```python
from build123d import *

# Parameters (mm, degrees)
SKETCH_R     = 16.037804
SKETCH_R_2   = 13.697081
PAD_DEPTH    = 50
POCKET_DEPTH = 18


with BuildPart() as part:
    # Sketch → Pad (new body)
    with BuildSketch(Plane.XZ):
        Circle(SKETCH_R)
        Circle(SKETCH_R_2, mode=Mode.SUBTRACT)
    extrude(amount=PAD_DEPTH)

    # Sketch001 → Pocket (cut)
    with BuildSketch(Plane.XY):
        Polygon((8.285895, -29.05966), (9.186356, -18.972051), (0.900461, -13.148425), (-8.285895, -17.412408), (-9.186356, -27.500017), (-0.900461, -33.323643), align=None)
    extrude(amount=-POCKET_DEPTH, mode=Mode.SUBTRACT)


solid = part.part
```
Geometry check sheet. Reference: the model listing, model coordinates, mm. A direction names the side the tool comes from. Give positions to 0.01 mm unless a question says otherwise; leave off trailing zeros. Loops run counter-clockwise (first coordinate to the right, second up) from the corner with the lowest first, then second, coordinate; pieces in that order, holes last. Notation, with made-up numbers: M 52,87 L 77,87 A19 ccw 77,99 Z; hole C 89.5,82 d11. An arc over 180 degrees is marked long. Write item = value, one per line. Start each with the question number.
1. Thickness scan on probe 1 along Z at (x, y) = (0, -36); probe 2 along Z at (x, y) = (0, -14); probe 3 along Y at (x, z) = (-1.5, -14). Record the ranges inside material, lowest first.
2. Section check D-D, the plane y = -39.5. Enter the section's corners in (x, z).
3. Section check A-A, the plane z = 0. Enter the section's corners in (x, y).
4. Section check C-C, the plane x = -13. Enter the section's corners in (y, z).
5. Draft check along Y on faces 1 (the face through (5.1, -16.1, -13.7)), 2 (the face through (12, -50, 7)), 3 (the face through (12, 0, 7)). Enter one of: +Y half, -Y half, draft (parallel to the pull), parting line (faces both ways), or undercut.
6. Tool access check on faces 4 (the face through (3.63, -31.22, -14.01)), 5 (the face through (-1.78, -24.65, 13.58)). Record the directions out of +Z, -Z, +X, -X, +Y, -Y that give a thin tool (end or side, any length) a straight path to the whole face; none if there is none.
7. Section check B-B, the plane x = 0. Enter the section's corners in (y, z).
8. Go/stop test with flat-tipped pins: P1, Ø5, axis at x = -0.5, z = 10.5, coming from the -Y side; P2, Ø6, axis at x = -12, y = -12, coming from the +Z side; P3, Ø12, axis at y = -23, z = -7.5, coming from the -X side; P4, Ø2, axis at y = -17, z = -7, coming from the +X side. Record where each tip stops, or that it passes through.
Values follow:
q1.probe_1 = -16.04 to -13.7, 13.7 to 16.04
q1.probe_2 = 13.7 to 16.04
q1.probe_3 = -50 to -32.9, -14.26 to 0
q2.outline = C 0,0 d32.08; hole C 0,0 d27.39
q3.outline = M -16.04,-50 L -13.7,-50 L -13.7,0 L -16.04,0 Z; M 13.7,-50 L 16.04,-50 L 16.04,0 L 13.7,0 Z
q4.outline = M -50,-9.39 L 0,-9.39 L 0,-4.31 L -50,-4.31 Z; M -50,4.31 L 0,4.31 L 0,9.39 L -50,9.39 Z
q5.face_1 = undercut
q5.face_2 = -Y half
q5.face_3 = +Y half
q6.face_4 = -Z
q6.face_5 = +Y, -Y
q7.outline = M -50,-16.04 L -32.91,-16.04 L -32.91,-13.7 L -50,-13.7 Z; M -50,13.7 L 0,13.7 L 0,16.04 L -50,16.04 Z; M -13.57,-16.04 L 0,-16.04 L 0,-13.7 L -13.57,-13.7 Z
q8.P1 = through
q8.P2 = 13.27
q8.P3 = -15.97
q8.P4 = 14.87
